Read the model definition and answer for the solid it produces. Units are mm, in the model's axes. Face numbers are marked on the shaded views. A direction names the side the tool comes from. Coordinates: 2 decimals unless noted, no trailing zeros. Order: outer loops, then holes, each group sorted by start corner. A loop starts at its lowest first (then second) coordinate and runs counter-clockwise, first axis right, second up. Notation, with made-up numbers: M 27.25,11 L 79.25,11 A23 ccw 79.25,25 Z; hole C 12.25,-4 d11. An arc over 180 degrees is marked long. Write each question's results on one line, items separated by ' | '.
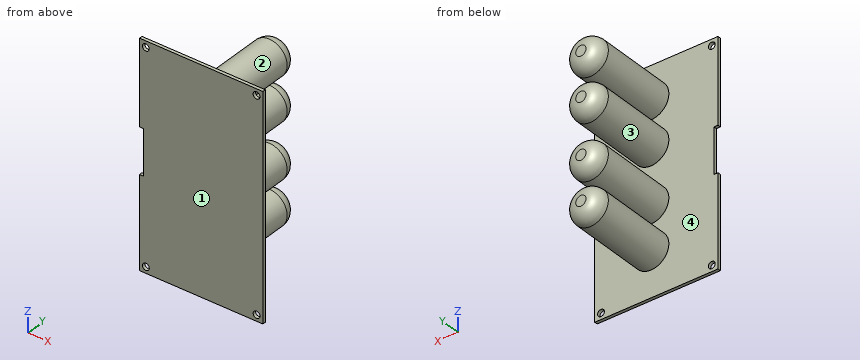
Autodesk Inventor part; units mm, degrees
ref_plane "YZ Plane" through (0, 0, 0) normal (1, 0, 0) x (0, 1, 0)
ref_plane "XZ Plane" through (0, 0, 0) normal (0, 1, 0) x (-1, 0, 0)
ref_plane "XY Plane" through (0, 0, 0) normal (0, 0, 1) x (1, 0, 0)
sketch "Sketch3" plane through (0, 0, 0) normal (0, 1, 0) x (-1, 0, 0)
  line L0 (0, 0) -> (62.23, 0)
  line L1 (62.23, 0) -> (62.23, -111.76)
  line L2 (62.23, -111.76) -> (0, -111.76)
  line L3 (0, -111.76) -> (0, 0)
  dimension "d53" = 62.23
  dimension "d54" = 111.76
extrude "Extrusion4" add sketch "Sketch3" along normal blind 1.5748
sketch "Sketch4" plane through (0, 1.5748, 0) normal (0, 1, 0) x (1, 0, 0)
  line L0 (-62.23, 0) -> (0, 0)
  line L1 (0, 0) -> (0, 111.76)
  line L2 (0, 111.76) -> (-62.23, 111.76)
  line L3 (-62.23, 111.76) -> (-62.23, 0)
  circle A0 centre (-59.055, 3.175) radius 1.7266
  circle A1 centre (-59.055, 108.585) radius 1.7266
  circle A2 centre (-3.175, 108.585) radius 1.7266
  circle A3 centre (-3.175, 3.175) radius 1.7266
  dimension "d57" = 3.4531
  dimension "d58" = 3.4531
  dimension "d59" = 3.4531
  dimension "d60" = 3.4531
  dimension "d61" = 3.175
  dimension "d62" = 3.175
  dimension "d63" = 3.175
  dimension "d64" = 3.175
  dimension "d65" = 3.175
  dimension "d66" = 3.175
  dimension "d67" = 3.175
  dimension "d68" = 3.175
extrude "Extrusion5" cut sketch "Sketch4" against normal blind 2.54 contours A0 | A1 | A2 | A3
sketch "Sketch5" plane through (0, 1.5748, 0) normal (0, 1, 0) x (1, 0, 0)
  circle A0 centre (-28.448, 17.272) radius 8.9535
  circle A1 centre (-28.448, 39.37) radius 8.9535
  circle A2 centre (-28.448, 67.31) radius 8.9535
  circle A3 centre (-28.448, 89.408) radius 8.9535
  line L0 (-62.23, 0) -> (0, 0)
  line L1 (0, 0) -> (0, 111.76)
  line L2 (-62.23, 111.76) -> (-62.23, 0)
  dimension "d71" = 17.907
  dimension "d72" = 17.907
  dimension "d73" = 17.907
  dimension "d74" = 17.907
  dimension "d75" = 17.272
  dimension "d78" = 22.098
  dimension "d80" = 27.94
  dimension "d82" = 22.098
  dimension "d86" = 33.782
extrude "Extrusion6" add sketch "Sketch5" along normal blind 45.72
fillet "Fillet2" radius 6.35 4 edges at (-37.4015, 47.2948, -17.272) (-37.4015, 47.2948, -39.37) (-37.4015, 47.2948, -67.31) (-37.4015, 47.2948, -89.408)
sketch "Sketch6" plane through (0, 1.5748, 0) normal (0, 1, 0) x (1, 0, 0)
  line L0 (-62.23, 111.76) -> (-62.23, 0)
  line L1 (-62.23, 0) -> (-62.23, 42.672)
  line L2 (-62.23, 42.672) -> (-60.198, 42.672)
  line L3 (-60.198, 42.672) -> (-60.198, 65.532)
  line L4 (-60.198, 65.532) -> (-62.23, 65.532)
  line L5 (-62.23, 42.672) -> (-62.23, 65.532)
  point P0 (0, 0)
  dimension "d87" = 42.672
  dimension "d88" = 2.032
  dimension "d89" = 22.86
extrude "Extrusion7" cut sketch "Sketch6" against normal blind 45.72
properties part number "PCB"
(1) Straight lines are drawn through the part: line 1 (Z direction, x = -31, y = 16); line 2 (Y direction, x = -5, z = -20.5); line 3 (Z direction, x = -36, y = 36). For each, find the intervals that lie inside material, in ascending order.
Conclusion:
line 1: -97.99 to -80.83, -75.89 to -58.73, -47.95 to -30.79, -25.85 to -8.69 | line 2: 0 to 1.57 | line 3: -94.22 to -84.6, -72.12 to -62.5, -44.18 to -34.56, -22.08 to -12.46
(2) For the marked faces 1 and 2, determine the directions among +Z, -Z, +X, -X, +Y, -Y from which every point of the face is accessible in a straight line to the end or side of a thin tool.
Conclusion:
face 1: +Z, -Z, +X, -X, -Y | face 2: +Y
(3) The part is cut by section D-D, the plane y = 43. Count the separate pieces of the cut face and the enclosed holes in it, then the cut area to 3 significant figures.
Conclusion:
separate pieces: 4 | enclosed holes: 0 | area: 932 mm²
(4) The part is cut by section B-B, the plane y = 31. Write down the section's boundary in (x, z).
Conclusion:
outline: C -28.45,-89.41 d17.91; C -28.45,-67.31 d17.91; C -28.45,-39.37 d17.91; C -28.45,-17.27 d17.91
(5) Given pin 1 (1.5 mm diameter, centred on y = 36.5, z = -83.5, fed in from +X); pin 2 (6 mm diameter, centred on y = 22, z = -81.5, fed in from -X); pin 3 (1 mm diameter, centred on y = 5.5, z = -73.5, fed in from +X), each flat-ended and moving along its own axis, determine where each tip first touches the part or whether it passes through.
Conclusion:
pin 1: x = -21.13 | pin 2: x = -35.94 | pin 3: x = -21.54
(6) The part is cut by section C-C, the plane z = -54. Write down the section's boundary in (x, y).
Conclusion:
outline: M -60.2,0 L 0,0 L 0,1.57 L -60.2,1.57 Z
(7) The mould has two halves that part along X. Classify the marked faces 3 and 4: pulls with the +X half, pulls with the -X half, needs draft (parallel to the pull), parting line crosses it, or undercut.
Conclusion:
face 3: parting line crosses it | face 4: needs draft
(8) The part is cut by section A-A, the plane x = -48. Write down the section's boundary in (y, z), then the cut area to 3 significant figures.
Conclusion:
outline: M 0,-111.76 L 1.57,-111.76 L 1.57,0 L 0,0 Z | area: 176 mm²
